Geometry: final body of the model. Coordinates: model frame, mm. Face numbers are marked on the shaded views. Give positions to 0.01 mm unless a question says otherwise; leave off trailing zeros. Order: outer loops, then holes, each group sorted by start corner. A loop starts at its lowest first (then second) coordinate and runs counter-clockwise, first axis right, second up. Notation, with made-up numbers: (-14.5, 48) -> (-7.5, 48) arc R28 cw to (-7.5, 68) -> close; hole circle Ø2 at (76.5, 69.5). An arc over 180 degrees is marked (long way). Answer in a Markdown table with one row per item. Add a question column.
Q1. Cut plane A-A on y = 36. Return the cut outline in (x, z), and give its area (3 significant figures).
Q2. Cut plane C-C on y = 71. Return the cut outline in (x, z), and give its area (3 significant figures).
Q3. Cut plane D-D on z = 7. Return the cut outline in (x, y), and give its area (3 significant figures).
Q4. Pull-direction query (Y, two-part tool) for the marked faces 1, 2 and 3; classes: +Y half, -Y half, draft (parallel to the pull), parting line (faces both ways), or undercut.
Q5. Contact query for flat-ended pins moving along their axis: P1, Ø3, axis at y = 51, z = 8, coming from the -X side; P2, Ø5, axis at y = 89.5, z = 2.5, coming from the -X side; P3, Ø3, axis at x = -8.5, z = 9, coming from the -Y side; P4, Ø1.5, axis at y = 77, z = 5.5, coming from the -X side. Output: stop coordinate, or through.
Q6. Cut plane B-B on x = -31. Return the cut outline in (y, z), and give its area (3 significant figures).
Q7. Line query: line 1 along Y through (x, z) = (0, 4.75); line 2 along Y through (x, z) = (12, 9); line 3 along X through (y, z) = (34, 3). Output: solid intervals per line, ascending. Write a range as from..to.
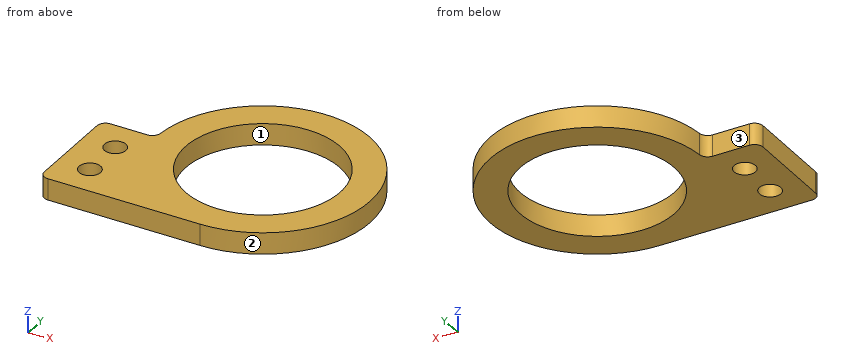
Autodesk Fusion 360 part; units mm, degrees
sketch "Sketch1" plane through (0, 0, 0) normal (0, 0, 1) x (1, 0, 0)
  line L0 (0, 0) -> (-75, 0)
  line L1 (-75, 0) -> (-75, 50)
  line L2 (-75, 50) -> (-50, 50)
  arc A0 (0, 0) -> (-50, 50) centre (0, 50) ccw
extrude "Extrude1" add sketch "Sketch1" along normal blind 10
fillet "Fillet1" radius 4 3 edges at (-75, 0, 5) (-75, 50, 5) (-50, 50, 5)
hole "Hole1" at (0, 50, 10) direction (0, 0, -1) diameter 72 depth 10 tip angle 118
hole "Hole2" at (-60.0592, 35.0034, 10) direction (0, 0, -1) diameter 10 depth 10 tip angle 118
hole "Hole3" at (-60.1262, 14.9013, 10) direction (0, 0, -1) diameter 10 depth 10 tip angle 118
Completed:
| question | item | result |
|---|---|---|
| 1 | outline | (-75, 0) -> (-64.96, 0) -> (-64.96, 10) -> (-75, 10) -> close; (-55.16, 0) -> (-33.17, 0) -> (-33.17, 10) -> (-55.16, 10) -> close; (33.17, 0) -> (48, 0) -> (48, 10) -> (33.17, 10) -> close |
| 1 | area | 469 mm² |
| 2 | outline | (-45.38, 0) -> (-29.24, 0) -> (-29.24, 10) -> (-45.38, 10) -> close; (29.24, 0) -> (45.38, 0) -> (45.38, 10) -> (29.24, 10) -> close |
| 2 | area | 323 mm² |
| 3 | outline | (-75, 4) arc R4 ccw to (-71, 0) -> (0, 0) arc R50 ccw (long way) to (-49.86, 53.7) arc R4 cw to (-53.85, 50) -> (-71, 50) arc R4 ccw to (-75, 46) -> close; hole circle Ø10 at (-60.13, 14.9); hole circle Ø10 at (-60.06, 35); hole circle Ø72 at (0, 50) |
| 3 | area | 5,410 mm² |
| 4 | face 1 | undercut |
| 4 | face 2 | parting line |
| 4 | face 3 | +Y half |
| 5 | P1 | stops at x = -72.94 |
| 5 | P2 | stops at x = -33.63 |
| 5 | P3 | stops at y = 0 |
| 5 | P4 | stops at x = -42.56 |
| 6 | outline | (0, 0) -> (31.7, 0) -> (31.7, 10) -> (0, 10) -> close; (68.3, 0) -> (89.23, 0) -> (89.23, 10) -> (68.3, 10) -> close |
| 6 | area | 526 mm² |
| 7 | line 1 | y = 0..14, 86..100 |
| 7 | line 2 | y = 1.46..16.06, 83.94..98.54 |
| 7 | line 3 | x = -75..-64.96, -55.16..-32.25, 32.25..47.37 |
